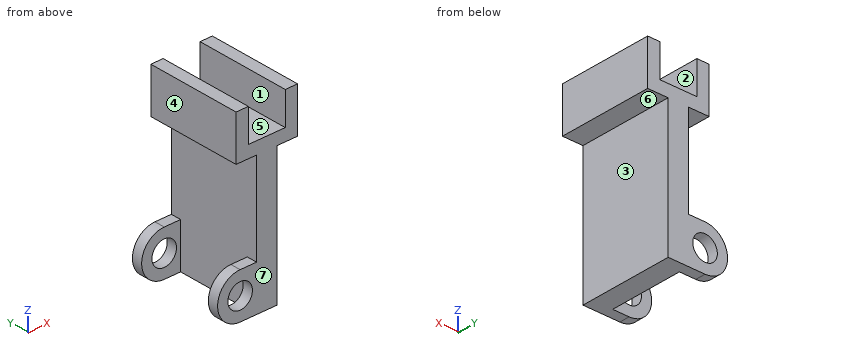
from build123d import *

# Parameters (mm, degrees)
F1_DEPTH = 116.84
F2_W     = 25.4
F2_H     = 116.84
F3_DEPTH = 170.18
F4_R     = 15.24
F5_DEPTH = 12.7


with BuildPart() as f1:
    # F0 (on Front) → F1 (new body)
    with BuildSketch(Plane.XZ):
        Polygon((-38.1, 86.1008339764), (0, 86.1008339764), (38.1, 86.1008339764), (38.1, 141.9808339764), (22.86, 141.9808339764), (22.86, 101.3408339764), (0, 101.3408339764), (-22.86, 101.3408339764), (-22.86, 141.9808339764), (-38.1, 141.9808339764), align=None)
    extrude(amount=F1_DEPTH)

    # F2 (on face) → F3 (join)
    with BuildSketch(Plane(origin=(0, 0, 86.1008339764), x_dir=(1, 0, 0), z_dir=(0, 0, -1))):
        with Locations((0, 58.42)):
            Rectangle(F2_W, F2_H)
    extrude(amount=F3_DEPTH)

    # F4 (on face) → F5 (join)
    with BuildSketch(Plane(origin=(0, 0, 0), x_dir=(-1, 0, 0), z_dir=(0, 1, 0))):
        with BuildLine():
            Line((12.7, -84.0791660236), (33.02, -84.0791660236))
            ThreePointArc((33.02, -84.0791660236), (60.96, -56.1391660236), (33.02, -28.1991660236))
            Line((33.02, -28.1991660236), (12.7, -28.1991660236))
            Line((12.7, -28.1991660236), (12.7, -84.0791660236))
        make_face()
        with Locations((33.02, -56.1391660236)):
            Circle(F4_R, mode=Mode.SUBTRACT)
    extrude(amount=-F5_DEPTH)

    # F7: F1 across plane


with BuildPart() as f1_1:
    add(f1.part)
    add(f1.part.mirror(Plane.XZ.offset(58.42)))


solid = f1_1.part
Build history of the part. All positions in model axes, mm. Face numbers are marked on the shaded views. A direction names the side the tool comes from. Coordinates: 2 decimals unless noted, no trailing zeros. Order: outer loops, then holes, each group sorted by start corner. A loop starts at its lowest first (then second) coordinate and runs counter-clockwise, first axis right, second up. Notation, with made-up numbers: (22, 38.5) -> (44, 38.5) arc R15 ccw to (44, 63.5) -> close; hole circle Ø4 at (79, -0.75). An arc over 180 degrees is marked (long way). One line per item, written item: value.
(1) Slice it at A-A, the plane y = -43. List the corners of the cut face in (x, z), plus the area to 3 significant figures.
Checked values:
outline: (-38.1, 86.1) -> (-12.7, 86.1) -> (-12.7, -84.08) -> (12.7, -84.08) -> (12.7, 86.1) -> (38.1, 86.1) -> (38.1, 141.98) -> (22.86, 141.98) -> (22.86, 101.34) -> (-22.86, 101.34) -> (-22.86, 141.98) -> (-38.1, 141.98) -> close
area: 6,720 mm2
(2) Probe line 1 (Z direction, x = -33.02, y = -2.75); line 2 (X direction, y = -56, z = 108); line 3 (Y direction, x = -32, z = -37). List the from-to ranges inside material, lowest first. Write a range as [from, to].
Checked values:
line 1: [-84.08, -71.38], [-40.9, -28.2], [86.1, 141.98]
line 2: [-38.1, -22.86], [22.86, 38.1]
line 3: [-116.84, -104.14], [-12.7, 0]
(3) Drop flat-ended pins along their axis: pin 1 Ø8 at (x, y) = (-18, -89) entering from +Z; pin 2 Ø4 at (y, z) = (-56, 118) entering from -X; pin 3 Ø14.5 at (x, z) = (-36.5, -53.5) entering from +Y; pin 4 Ø7.5 at (x, y) = (-25.5, -61) entering from -Z. Give the stop position or say it passes through.
Checked values:
pin 1: z = 101.34
pin 2: x = -38.1
pin 3: through
pin 4: z = 86.1
(4) Slice it at C-C, the plane x = -52. List the corners of the cut face in (y, z), plus the area to 3 significant figures.
Checked values:
outline: (-116.84, -76.64) -> (-104.14, -76.64) -> (-104.14, -35.64) -> (-116.84, -35.64) -> close; (-12.7, -76.64) -> (0, -76.64) -> (0, -35.64) -> (-12.7, -35.64) -> close
area: 1,040 mm2
(5) Tool access for the marked faces 5, 6 and 7: list every direction of +Z, -Z, +X, -X, +Y, -Y with a clear straight run to the whole face (end or side of a thin tool).
Checked values:
face 5: +Z, +Y, -Y
face 6: -Z, +X, +Y, -Y
face 7: +Z, -Z, +X, -X, -Y
(6) Mould opens along X. For the marked faces 1, 2, 3 and 4 say: pulls with the +X half, pulls with the -X half, needs draft (parallel to the pull), parting line crosses it, or undercut.
Checked values:
face 1: undercut
face 2: undercut
face 3: pulls with the +X half
face 4: pulls with the -X half
(7) Slice it at D-D, the plane x = 5. List the corners of the cut face in (y, z).
Checked values:
outline: (-116.84, -84.08) -> (0, -84.08) -> (0, 101.34) -> (-116.84, 101.34) -> close
(8) Slice it at B-B, the plane z = 120. List the corners of the cut face in (x, y), plus the area to 3 significant figures.
Checked values:
outline: (-38.1, -116.84) -> (-22.86, -116.84) -> (-22.86, 0) -> (-38.1, 0) -> close; (22.86, -116.84) -> (38.1, -116.84) -> (38.1, 0) -> (22.86, 0) -> close
area: 3,560 mm2
